The drawing under review shows one solid part. Ordinate dimensions are in mm from its lowest x, y, z. Coordinates: 2 decimals unless noted, no trailing zeros. Write each loop counter-clockwise with the first axis right and the second up, starting at its lowest first coordinate (ties: lowest second). Pieces come first, ordered by that corner, then holes. Notation, with made-up numbers: (23.5, 80) -> (76.5, 80) arc R32 cw to (76.5, 118) -> close; hole circle Ø11 at (8, 9.5). An arc over 180 degrees is marked (long way). One line per question, with ' | ' between items. Start each with the question number.
Q1. Add section B-B on z = 6.25. State the section outline as (x, y) points.
Q2. Draft analysis for pull direction Y (two halves, no side actions). For the marked faces 1, 2 and 3, state which applies: pulls with the +Y half, pulls with the -Y half, needs draft (parallel to the pull), parting line crosses it, or undercut.
Q3. Wall thickness on probe 1 along X at (y, z) = (11.5, 4); probe 2 along X at (y, z) = (13.75, 3.5); probe 3 along Y at (x, z) = (17, 3): over which ranges is each line inside the solid? List them lowest first.
Q4. Add section A-A on y = 11.5. State the section outline as (x, z) points.
Q5. For P1, Ø3.5, axis at x = 50, y = 11.5, coming from the +Z side; P2, Ø2, axis at x = 36, z = 3, coming from the +Y side; P3, Ø0.6, axis at x = 55, y = 1, coming from the -Z side; P4, Ø2, axis at x = 29, z = 2.5, coming from the -Y side, all flat-tipped, find the tip position at first contact; note any pin that passes through.
Q6. Add section C-C on x = 70. State the section outline as (y, z) points.
Q7. Add section D-D on x = 17.5. State the section outline as (y, z) points, and give its area (3 significant figures).
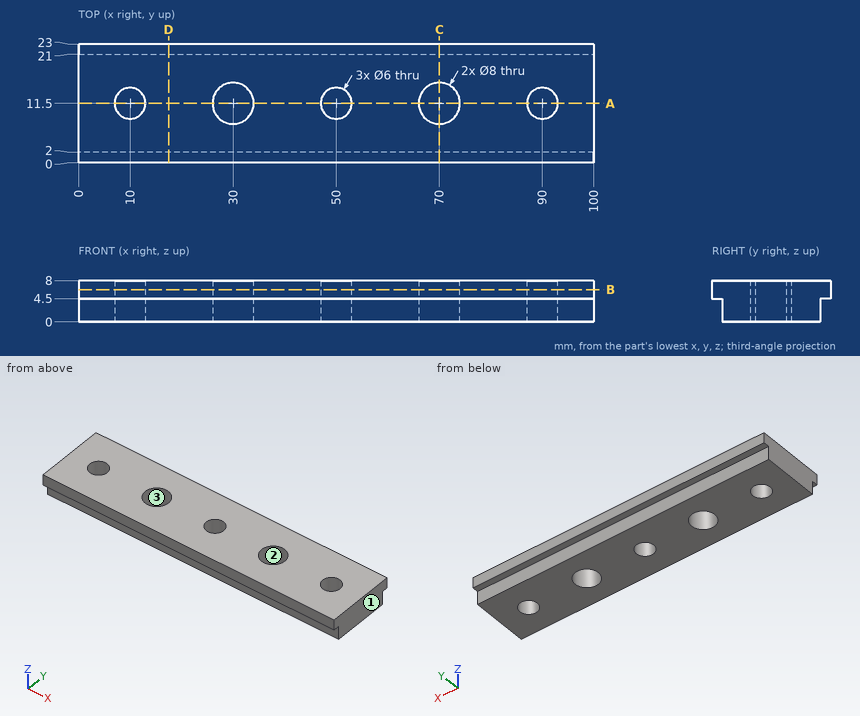
Output values:
1) outline: (0, 0) -> (100, 0) -> (100, 23) -> (0, 23) -> close; hole circle Ø6 at (10, 11.5); hole circle Ø8 at (30, 11.5); hole circle Ø6 at (50, 11.5); hole circle Ø8 at (70, 11.5); hole circle Ø6 at (90, 11.5)
2) face 1: needs draft | face 2: undercut | face 3: undercut
3) probe 1: x = 0 to 7, 13 to 26, 34 to 47, 53 to 66, 74 to 87, 93 to 100 | probe 2: x = 0 to 8.02, 11.98 to 26.69, 33.31 to 48.02, 51.98 to 66.69, 73.31 to 88.02, 91.98 to 100 | probe 3: y = 2 to 21
4) outline: (0, 0) -> (7, 0) -> (7, 8) -> (0, 8) -> close; (13, 0) -> (26, 0) -> (26, 8) -> (13, 8) -> close; (34, 0) -> (47, 0) -> (47, 8) -> (34, 8) -> close; (53, 0) -> (66, 0) -> (66, 8) -> (53, 8) -> close; (74, 0) -> (87, 0) -> (87, 8) -> (74, 8) -> close; (93, 0) -> (100, 0) -> (100, 8) -> (93, 8) -> close
5) P1: passes through | P2: stops at y = 21 | P3: stops at z = 4.5 | P4: stops at y = 2
6) outline: (0, 4.5) -> (2, 4.5) -> (2, 0) -> (7.5, 0) -> (7.5, 8) -> (0, 8) -> close; (15.5, 0) -> (21, 0) -> (21, 4.5) -> (23, 4.5) -> (23, 8) -> (15.5, 8) -> close
7) outline: (0, 4.5) -> (2, 4.5) -> (2, 0) -> (21, 0) -> (21, 4.5) -> (23, 4.5) -> (23, 8) -> (0, 8) -> close | area: 166 mm2
